```python
from build123d import *

# Parameters (mm, degrees)
F0_R     = 8.1762348774
F1_DEPTH = 16.764


with BuildPart() as f1:
    # F0 (on Front) → F1 (new body)
    with BuildSketch(Plane.XZ):
        with BuildLine():
            ThreePointArc((10.7045995524, -2.0546407042), (10.8510399299, -1.0319556383), (10.9, 0))
            ThreePointArc((10.9, 0), (8.8812984176, 6.3192197633), (3.5729287307, 10.2977755018))
            ThreePointArc((3.5729287307, 10.2977755018), (0, 10.9), (-3.5729287307, 10.2977755018))
            ThreePointArc((-3.5729287307, 10.2977755018), (-9.4396769013, 5.45), (-10.7045995524, -2.0546407042))
            ThreePointArc((-10.7045995524, -2.0546407042), (-9.4396769013, -5.45), (-7.1316708216, -8.2431347976))
            ThreePointArc((-7.1316708216, -8.2431347976), (0, -10.9), (7.1316708216, -8.2431347976))
            ThreePointArc((7.1316708216, -8.2431347976), (9.4396769013, -5.45), (10.7045995524, -2.0546407042))
        make_face()
        Circle(F0_R, mode=Mode.SUBTRACT)
        with BuildLine():
            ThreePointArc((-3.5729287307, 10.2977755018), (0, 10.9), (3.5729287307, 10.2977755018))
            Line((3.5729287307, 10.2977755018), (3.5729287307, 19.8155592292))
            Line((3.5729287307, 19.8155592292), (5.078934896, 22.8855756019))
            Line((5.078934896, 22.8855756019), (5.3861358478, 25.1383827151))
            ThreePointArc((5.3861358478, 25.1383827151), (4.8979120469, 28.5734299473), (2.6770923706, 31.239114087))
            Line((2.6770923706, 31.239114087), (0.2394953625, 32.9048861241))
            ThreePointArc((0.2394953625, 32.9048861241), (0.1250583953, 32.9655378852), (0, 32.9992254696))
            ThreePointArc((0, 32.9992254696), (-0.1387115468, 33.0035052248), (-0.2744548515, 32.9746440958))
            Line((-0.2744548515, 32.9746440958), (-2.6277035917, 32.1694766202))
            ThreePointArc((-2.6277035917, 32.1694766202), (-5.7380801108, 29.853914456), (-6.9220383964, 26.1614203118))
            Line((-6.9220383964, 26.1614203118), (-6.9220383964, 25.6764997761))
            Line((-6.9220383964, 25.6764997761), (-3.5729287307, 19.8155592292))
            Line((-3.5729287307, 19.8155592292), (-3.5729287307, 10.2977755018))
        make_face()
        Polygon((-1.8806647364, 30.2667208016), (0, 30.2667208016), (1.8806647364, 30.2667208016), (3.7613294728, 27.0093139261), (1.8806647364, 23.7519070506), (0, 23.7519070506), (-1.8806647364, 23.7519070506), (-3.7613294728, 27.0093139261), align=None, mode=Mode.SUBTRACT)
        with BuildLine():
            Line((18.947242048, -6.8135325679), (10.7045995524, -2.0546407042))
            ThreePointArc((10.7045995524, -2.0546407042), (9.4396769013, -5.45), (7.1316708216, -8.2431347976))
            Line((7.1316708216, -8.2431347976), (15.3743133173, -13.0020266613))
            Line((15.3743133173, -13.0020266613), (17.2800224035, -15.8412744451))
            Line((17.2800224035, -15.8412744451), (19.4543915529, -17.5257716809))
            ThreePointArc((19.4543915529, -17.5257716809), (22.2820714904, -18.6631064405), (25.2854497533, -18.1444319823))
            Line((25.2854497533, -18.1444319823), (26.7438602666, -17.4440315112))
            ThreePointArc((26.7438602666, -17.4440315112), (27.5677621083, -16.9572968799), (28.2963483866, -16.3369043581))
            ThreePointArc((28.2963483866, -16.3369043581), (28.5524118785, -16.0596668899), (28.7891431297, -15.7657494859))
            Line((28.7891431297, -15.7657494859), (29.2797580155, -13.2677285991))
            ThreePointArc((29.2797580155, -13.2677285991), (28.8843269769, -9.8844337919), (26.595254614, -7.3618959476))
            Line((26.595254614, -7.3618959476), (26.3302729622, -7.2089087196))
            ThreePointArc((26.3302729622, -7.2089087196), (25.3589284831, -6.933455194), (24.3538425846, -6.8376059446))
            Line((24.3538425846, -6.8376059446), (18.947242048, -6.8135325679))
        make_face()
        Polygon((25.9469195413, -14.9804609818), (25.5060197939, -15.7441217452), (21.5879713963, -15.7441217452), (19.6289471975, -12.3509922996), (20.0698469448, -11.5873315362), (21.5879713963, -8.957862854), (25.5060197939, -8.957862854), (27.4650439927, -12.3509922996), align=None, mode=Mode.SUBTRACT)
        with BuildLine():
            ThreePointArc((-7.1316708216, -8.2431347976), (-9.4396769013, -5.45), (-10.7045995524, -2.0546407042))
            Line((-10.7045995524, -2.0546407042), (-18.947242048, -6.8135325679))
            Line((-18.947242048, -6.8135325679), (-22.3589572995, -7.0443011568))
            Line((-22.3589572995, -7.0443011568), (-24.904959273, -8.0851114596))
            ThreePointArc((-24.904959273, -8.0851114596), (-27.3037600362, -9.9652867393), (-28.3562639105, -12.8256258414))
            Line((-28.3562639105, -12.8256258414), (-28.621501234, -16.3145697088))
            ThreePointArc((-28.621501234, -16.3145697088), (-28.6179368344, -16.4128846333), (-28.5926007189, -16.5079457219))
            ThreePointArc((-28.5926007189, -16.5079457219), (-28.5427339525, -16.6008192319), (-28.4721935743, -16.6791533769))
            Line((-28.4721935743, -16.6791533769), (-26.5457321837, -18.3603963741))
            ThreePointArc((-26.5457321837, -18.3603963741), (-22.9852082659, -19.8962803729), (-19.1954353909, -19.0753712531))
            Line((-19.1954353909, -19.0753712531), (-18.7754818882, -18.8329109853))
            Line((-18.7754818882, -18.8329109853), (-15.3743133173, -13.0020266613))
            Line((-15.3743133173, -13.0020266613), (-7.1316708216, -8.2431347976))
        make_face()
        Polygon((-19.1541526712, -11.0586552008), (-18.5637420285, -11.5622606176), (-19.2950824343, -15.5223581541), (-23.0902977052, -16.8690475522), (-25.5637619278, -14.7592448305), (-26.1541725704, -14.2556394138), (-25.4228321647, -10.2955418772), (-21.6276168938, -8.9488524791), align=None, mode=Mode.SUBTRACT)
        with BuildLine():
            ThreePointArc((28.7891431297, -15.7657494859), (29.6901919838, -10.8751191131), (26.3302729622, -7.2089087196))
            Line((26.3302729622, -7.2089087196), (26.595254614, -7.3618959476))
            ThreePointArc((26.595254614, -7.3618959476), (28.8843269769, -9.8844337919), (29.2797580155, -13.2677285991))
            Line((29.2797580155, -13.2677285991), (28.7891431297, -15.7657494859))
        make_face()
        with BuildLine():
            Line((28.6382036926, -16.534274611), (28.7891431297, -15.7657494859))
            ThreePointArc((28.7891431297, -15.7657494859), (28.5524118785, -16.0596668899), (28.2963483866, -16.3369043581))
            Line((28.2963483866, -16.3369043581), (28.6382036926, -16.534274611))
        make_face()
    extrude(amount=-F1_DEPTH)


solid = f1.part
```
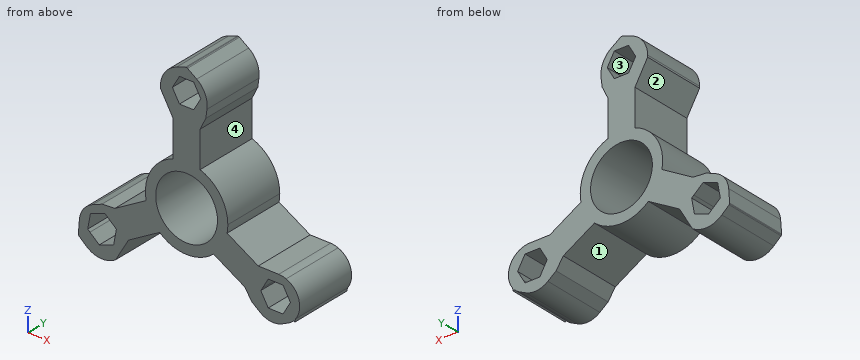
For this review, take the finished solid that the model builds, in its own axes (mm). Face numbers are marked on the shaded views. A direction names the side the tool comes from. Round coordinates to 2 decimals unless told otherwise and drop trailing zeros. Write each loop counter-clockwise with the first axis right and the second up, starting at its lowest first coordinate (ties: lowest second). Pieces come first, ordered by that corner, then holes. Notation, with made-up numbers: (8.25, 40.25) - (38.25, 40.25) arc R16 cw to (38.25, 70.25) - close; hole circle Ø4 at (84, 74). An arc over 180 degrees is marked (long way). Answer as a JSON object with one key per item and string values.
1. To check wall thickness, follow line 1 along X through (y, z) = (6.5, -11); line 2 along Z through (x, y) = (-4.5, 2.25); line 3 along X through (y, z) = (11.75, -12). State the ranges of each line that lie inside material, in increasing order.
Response values:
{"line 1": "x = -27.9 to -25.55, -19.22 to -11.91, 11.91 to 20.41, 26.69 to 29.72", "line 2": "z = -9.93 to -6.83, 6.83 to 9.93, 21.44 to 31.15", "line 3": "x = -28.23 to -25.74, -18.64 to -13.64, 13.64 to 19.83, 27.26 to 29.89"}
2. For pin 1 Ø1 at (y, z) = (8.5, 3.5) entering from +X; pin 2 Ø14.5 at (x, z) = (0, 0) entering from +Y; pin 3 Ø5 at (y, z) = (5, 14) entering from +X; pin 4 Ø1.1 at (x, y) = (0, 10.5) entering from -Z, all flat-tipped, find the tip position at first contact; note any pin that passes through.
Response values:
{"pin 1": "stops at x = 10.48", "pin 2": "passes through", "pin 3": "stops at x = 3.57", "pin 4": "stops at z = -10.9"}
3. We need section C-C on z = 1. Give the boundary of the cut face in (x, y).
Response values:
{"outline": "(-10.85, 0) - (-8.11, 0) - (-8.11, 16.76) - (-10.85, 16.76) - close; (8.11, 0) - (10.85, 0) - (10.85, 16.76) - (8.11, 16.76) - close"}
4. We need section D-D on x = -14.5. Give the boundary of the cut face in (y, z).
Response values:
{"outline": "(0, -12.5) - (16.76, -12.5) - (16.76, -4.25) - (0, -4.25) - close"}
5. Tool access review of the marked faces 1, 2, 3 and 4: name each direction out of +Z, -Z, +X, -X, +Y, -Y from which nothing blocks a thin tool from reaching the whole face with its end or side.
Response values:
{"face 1": "-Z, +Y, -Y", "face 2": "-X, +Y, -Y", "face 3": "+Y, -Y", "face 4": "+X, +Y, -Y"}
6. We need section A-A on x = -20.5. Give the boundary of the cut face in (y, z), then the cut area to 3 significant figures.
Response values:
{"outline": "(0, -19.64) - (16.76, -19.64) - (16.76, -15.95) - (0, -15.95) - close; (0, -9.91) - (16.76, -9.91) - (16.76, -6.92) - (0, -6.92) - close", "area": "112 mm2"}
7. We need section B-B on y = 8.25. Count the separate pieces of the cut face and the enclosed holes in it, then the cut area to 3 significant figures.
Response values:
{"separate pieces": "1", "enclosed holes": "4", "area": "624 mm2"}
